```python
from build123d import *
from build123d.topology import SkipClean

# Parameters (mm, degrees)
BOSS_EXTRUDE2_DEPTH     = 34
CUT_EXTRUDE3_DEPTH      = 110.79981785
CUT_EXTRUDE3_DEPTH_BACK = 110.79981785
SKETCH3_W               = 22
SKETCH3_H               = 15
SKETCH3_W_2             = 6


with BuildPart() as part:
    # Sketch1 → Boss-Extrude2 (new body)
    # profile 1 of 2: a face of its own
    with SkipClean():  # the faces are left unmerged after this step: merging them gives an invalid solid
        with BuildSketch(Plane.XY):
            with BuildLine():
                Line((-15, 0), (-15, -85))
                ThreePointArc((-15, -85), (0, -100), (15, -85))
                Line((15, -85), (15, 0))
                ThreePointArc((15, 0), (0, 15), (-15, 0))
            make_face()
            with BuildLine():
                ThreePointArc((-10.25, -85), (0, -95.25), (10.25, -85))
                Line((10.25, -85), (10.25, 0))
                ThreePointArc((10.25, 0), (0, 10.25), (-10.25, 0))
                Line((-10.25, 0), (-10.25, -85))
            make_face(mode=Mode.SUBTRACT)
        # profile 2 of 2: a face of its own
        with BuildSketch(Plane.XY):
            with BuildLine():
                Line((10.25, -85), (10.25, 0))
                ThreePointArc((10.25, 0), (0, -10.25), (-10.25, 0))
                Line((-10.25, 0), (-10.25, -85))
                ThreePointArc((-10.25, -85), (0, -74.75), (10.25, -85))
            make_face()
        extrude(amount=BOSS_EXTRUDE2_DEPTH)
    add(part.part.scale(1), mode=Mode.REPLACE)  # the faces are merged on a copy

    # Sketch3 → Cut-Extrude3 (cut, two sides: drawn at the far end of the back side and taken through both)
    with BuildSketch(Plane.ZY.offset(15).offset(-CUT_EXTRUDE3_DEPTH_BACK)):
        with Locations((17, -77.5)):
            Rectangle(SKETCH3_W, SKETCH3_H)
        with Locations((17, -92.5)):
            Rectangle(SKETCH3_W, SKETCH3_H)
        with Locations((3, -7.5)):
            Rectangle(SKETCH3_W_2, SKETCH3_H)
        with Locations((31, -7.5)):
            Rectangle(SKETCH3_W_2, SKETCH3_H)
        with Locations((31, 7.5)):
            Rectangle(SKETCH3_W_2, SKETCH3_H)
        with Locations((3, 7.5)):
            Rectangle(SKETCH3_W_2, SKETCH3_H)
    extrude(amount=CUT_EXTRUDE3_DEPTH + CUT_EXTRUDE3_DEPTH_BACK, mode=Mode.SUBTRACT)


solid = part.part
```
The listing builds one solid part. Answer for the finished solid, in the listing's coordinates (mm). A direction names the side the tool comes from. Round coordinates to 2 decimals unless told otherwise and drop trailing zeros. Loops run counter-clockwise (first coordinate to the right, second up) from the corner with the lowest first, then second, coordinate; pieces in that order, holes last.
Q1. Given pin 1 Ø1 at (x, z) = (8, 30) entering from +Y; pin 2 Ø8 at (x, z) = (10, 26.5) entering from +Y; pin 3 Ø5 at (x, z) = (-6, 7.5) entering from -Y, each flat-ended and moving along its own axis, determine where each tip first touches the part or whether it passes through.
Q2. Section C-C, the plane y = 8.5 is taken. Determine the outline of the cut face in (x, z).
Q3. Section A-A, the plane x = 0 is taken. Determine the outline of the cut face in (y, z).
Q4. Section B-B, the plane z = 10 is taken. Determine the outline of the cut face in (x, y).
Q5. Which of the six approach directions +Z, -Z, +X, -X, +Y, -Y give full straight-line access (tool end or side, diameter ignored) to faces 1 (the face through (0, -100, 3)), 2 (the face through (0, -15, 3)), 3 (the face through (-3, -10, 28)), 4 (the face through (-3, -75, 28)), 5 (the face through (0, 15, 17))?
Q6. For a pull along Z with two mould halves and no side action, classify faces 6 (the face through (0, -15, 31)), 7 (the face through (-3, -10, 6)), 8 (the face through (0, -70, 17)) as released by +Z, released by -Z, zero draft, split by the parting line, or undercut.
Q7. Find the intervals of material crossed by line 1 (X direction, y = 0.5, z = 15); line 2 (Z direction, x = 11.5, y = -73.5); line 3 (Z direction, x = -11, y = -11), in increasing order.
Q8. Section D-D, the plane y = -92.5 is taken. Determine the outline of the cut face in (x, z), then the cut area to 3 significant figures.
Completed:
1. pin 1: stops at y = -15
1. pin 2: stops at y = 13.75
1. pin 3: stops at y = -99.46
2. outline: (-12.36, 6) - (-5.73, 6) - (-5.73, 28) - (-12.36, 28) - close; (5.73, 6) - (12.36, 6) - (12.36, 28) - (5.73, 28) - close
3. outline: (-100, 0) - (-95.25, 0) - (-95.25, 6) - (-100, 6) - close; (-100, 28) - (-95.25, 28) - (-95.25, 34) - (-100, 34) - close; (-74.75, 0) - (-15, 0) - (-15, 6) - (-10.25, 6) - (-10.25, 28) - (-15, 28) - (-15, 34) - (-74.75, 34) - (-74.75, 28) - (-70, 28) - (-70, 6) - (-74.75, 6) - close; (10.25, 6) - (15, 6) - (15, 28) - (10.25, 28) - close
4. outline: (-15, -70) - (15, -70) - (15, 0) arc R15 ccw to (-15, 0) - close; hole circle Ø20.5 at (0, 0)
5. face 1: +Z, -Z, -Y
5. face 2: -Z, +X, -X, +Y
5. face 3: +Z, +X, -X, +Y
5. face 4: +X, -X, -Y
5. face 5: +Z, -Z, +Y
6. face 6: zero draft
6. face 7: released by -Z
6. face 8: undercut
7. line 1: x = -14.99 to -10.24, 10.24 to 14.99
7. line 2: z = 0 to 6, 28 to 34
7. line 3: z = 6 to 28
8. outline: (-12.99, 0) - (-6.99, 0) - (-6.99, 6) - (-12.99, 6) - close; (-12.99, 28) - (-6.99, 28) - (-6.99, 34) - (-12.99, 34) - close; (6.99, 0) - (12.99, 0) - (12.99, 6) - (6.99, 6) - close; (6.99, 28) - (12.99, 28) - (12.99, 34) - (6.99, 34) - close
8. area: 144 mm2
